Design review of the part built by this model. Coordinates are the model's own, in mm. Face numbers are marked on the shaded views. A direction names the side the tool comes from. Give positions to 0.01 mm unless a question says otherwise; leave off trailing zeros. Write each loop counter-clockwise with the first axis right and the second up, starting at its lowest first coordinate (ties: lowest second). Pieces come first, ordered by that corner, then holes. Notation, with made-up numbers: (17, -31.5) -> (42, -31.5) arc R34 ccw to (42, 6.5) -> close; hole circle Ø4 at (-4.75, -26). An arc over 180 degrees is marked (long way). Return JSON: item names as keys, results as strings. Group by question number.
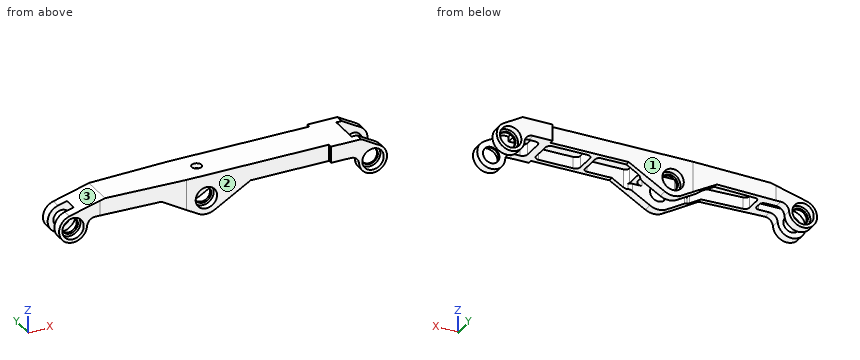
from build123d import *

# Parameters (mm, degrees)
F0_R                   = 5
F1_DEPTH               = 14
F2_W                   = 220
F2_H                   = 50
F3_DEPTH               = 25
F5_DEPTH               = 25
F5_DEPTH_BACK          = 7
F7_DEPTH               = 25
F7_DEPTH_BACK          = 4
F9_DEPTH               = 4
F9_DEPTH_BACK          = 4
F12_DEPTH              = 12
F13_R                  = 2.5
F14_D                  = 6
F18_D                  = 1
F18_DEPTH              = 12
F18_CBORE_D            = 13
F18_CBORE_DEPTH        = 4
F18_TIP                = 0.3004303095
F18_ON_F16_D           = 1
F18_ON_F16_DEPTH       = 12
F18_ON_F16_CBORE_D     = 13
F18_ON_F16_CBORE_DEPTH = 4
F18_ON_F16_TIP         = 0.3004303095
F18_ON_F17_D           = 1
F18_ON_F17_DEPTH       = 12
F18_ON_F17_CBORE_D     = 13
F18_ON_F17_CBORE_DEPTH = 4
F18_ON_F17_TIP         = 0.3004303095
F22_D                  = 1
F22_DEPTH              = 12
F22_CBORE_D            = 13
F22_CBORE_DEPTH        = 4
F22_TIP                = 0.3004303095
F22_ON_F20_D           = 1
F22_ON_F20_DEPTH       = 12
F22_ON_F20_CBORE_D     = 13
F22_ON_F20_CBORE_DEPTH = 4
F22_ON_F20_TIP         = 0.3004303095
F22_ON_F21_D           = 1
F22_ON_F21_DEPTH       = 12
F22_ON_F21_CBORE_D     = 13
F22_ON_F21_CBORE_DEPTH = 4
F22_ON_F21_TIP         = 0.3004303095


with BuildPart() as f1:
    # F0 (on Front) → F1 (new body, symmetric)
    with BuildSketch(Plane.XZ):
        with BuildLine():
            Line((92.751288694, 14), (-60.5927667879, 14))
            Line((-60.5927667879, 14), (-82.1999618834, 8.2103695235))
            ThreePointArc((-82.1999618834, 8.2103695235), (-85.4208481231, -6.5470913868), (-71.5233516925, -0.6296296296))
            ThreePointArc((-71.5233516925, -0.6296296296), (-69.9391570694, 2.664140544), (-66.5370879822, 4))
            Line((-66.5370879822, 4), (-26.9282032303, 4))
            Line((-26.9282032303, 4), (-5, -8.6602540378))
            ThreePointArc((-5, -8.6602540378), (0, -10), (5, -8.6602540378))
            Line((5, -8.6602540378), (26.9282032303, 4))
            Line((26.9282032303, 4), (86.5370879822, 4))
            ThreePointArc((86.5370879822, 4), (89.9391570694, 2.664140544), (91.5233516925, -0.6296296296))
            ThreePointArc((91.5233516925, -0.6296296296), (104.5199051071, -7.1986427765), (104.25, 7.3612159322))
            Line((104.25, 7.3612159322), (92.751288694, 14))
        make_face()
        with Locations((-80, 0)):
            Circle(F0_R, mode=Mode.SUBTRACT)
        Circle(F0_R, mode=Mode.SUBTRACT)
        with Locations((100, 0)):
            Circle(F0_R, mode=Mode.SUBTRACT)
    extrude(amount=F1_DEPTH, both=True)

    # F2 (on face) → F3 (cut)
    with BuildSketch(Plane.XY.offset(14)):
        with Locations((10, 0)):
            Rectangle(F2_W, F2_H)
        Polygon((-63.5, -9.5), (-88.5, -9.5), (-88.5, 9.5), (-63.5, 9.5), (-12, 11.5), (74.5, 11.5), (74.5, 14), (108.5, 14), (108.5, 9), (89.5, 9), (89.5, -9), (108.5, -9), (108.5, -14), (74.5, -14), (74.5, -11.5), (-12, -11.5), align=None, mode=Mode.SUBTRACT)
    extrude(amount=-F3_DEPTH, mode=Mode.SUBTRACT)

    # F4 (on face) → F5 (cut, two sides)
    with BuildSketch(Plane(origin=(0, 0, 4), x_dir=(1, 0, 0), z_dir=(0, 0, -1))) as f5_sk:
        with BuildLine():
            ThreePointArc((74.5, 5.5), (73.6213203436, 7.6213203436), (71.5, 8.5))
            Line((71.5, 8.5), (50.5, 8.5))
            ThreePointArc((50.5, 8.5), (48.3786796564, 7.6213203436), (47.5, 5.5))
            Line((47.5, 5.5), (47.5, -5.5))
            ThreePointArc((47.5, -5.5), (48.3786796564, -7.6213203436), (50.5, -8.5))
            Line((50.5, -8.5), (71.5, -8.5))
            ThreePointArc((71.5, -8.5), (73.6213203436, -7.6213203436), (74.5, -5.5))
            Line((74.5, -5.5), (74.5, 5.5))
        make_face()
        with BuildLine():
            Line((44.5, -6), (44.5, 6))
            ThreePointArc((44.5, 6), (43.767766953, 7.767766953), (42, 8.5))
            Line((42, 8.5), (20, 8.5))
            ThreePointArc((20, 8.5), (18.232233047, 7.767766953), (17.5, 6))
            Line((17.5, 6), (17.5, -6))
            ThreePointArc((17.5, -6), (18.232233047, -7.767766953), (20, -8.5))
            Line((20, -8.5), (42, -8.5))
            ThreePointArc((42, -8.5), (43.767766953, -7.767766953), (44.5, -6))
        make_face()
        with BuildLine():
            Line((89.5, -9), (89.5, 9))
            Line((89.5, 9), (82.5, 9))
            ThreePointArc((82.5, 9), (80.3786796564, 8.1213203436), (79.5, 6))
            Line((79.5, 6), (79.5, -6))
            ThreePointArc((79.5, -6), (80.3786796564, -8.1213203436), (82.5, -9))
            Line((82.5, -9), (89.5, -9))
        make_face()
        with BuildLine():
            Line((-17.5, -5.6851745289), (-17.5, 5.6851745289))
            ThreePointArc((-17.5, 5.6851745289), (-18.2668721376, 7.4869147467), (-20.09701425, 8.1832914668))
            Line((-20.09701425, 8.1832914668), (-52.09701425, 6.9405730202))
            ThreePointArc((-52.09701425, 6.9405730202), (-53.8017402178, 6.1755839447), (-54.5, 4.4424560823))
            Line((-54.5, 4.4424560823), (-54.5, -4.4424560823))
            ThreePointArc((-54.5, -4.4424560823), (-53.8017402178, -6.1755839447), (-52.09701425, -6.9405730202))
            Line((-52.09701425, -6.9405730202), (-20.09701425, -8.1832914668))
            ThreePointArc((-20.09701425, -8.1832914668), (-18.2668721376, -7.4869147467), (-17.5, -5.6851745289))
        make_face()
        with BuildLine():
            Line((-14.5, 1.5), (-14.5, -1.5))
            ThreePointArc((-14.5, -1.5), (-13.1819805153, -4.6819805153), (-10, -6))
            Line((-10, -6), (10, -6))
            ThreePointArc((10, -6), (13.1819805153, -4.6819805153), (14.5, -1.5))
            Line((14.5, -1.5), (14.5, 1.5))
            ThreePointArc((14.5, 1.5), (13.1819805153, 4.6819805153), (10, 6))
            Line((10, 6), (-10, 6))
            ThreePointArc((-10, 6), (-13.1819805153, 4.6819805153), (-14.5, 1.5))
        make_face()
    extrude(amount=F5_DEPTH, mode=Mode.SUBTRACT)
    extrude(f5_sk.sketch, amount=-F5_DEPTH_BACK, mode=Mode.SUBTRACT)

    # F6 (on face) → F7 (cut, two sides)
    with BuildSketch(Plane(origin=(0, 0, 4), x_dir=(1, 0, 0), z_dir=(0, 0, -1))) as f7_sk:
        with BuildLine():
            Line((-88.5, 4), (-88.5, -4))
            Line((-88.5, -4), (-60, -4))
            ThreePointArc((-60, -4), (-58.232233047, -3.267766953), (-57.5, -1.5))
            Line((-57.5, -1.5), (-57.5, 1.5))
            ThreePointArc((-57.5, 1.5), (-58.232233047, 3.267766953), (-60, 4))
            Line((-60, 4), (-88.5, 4))
        make_face()
    extrude(amount=F7_DEPTH, mode=Mode.SUBTRACT)
    extrude(f7_sk.sketch, amount=-F7_DEPTH_BACK, mode=Mode.SUBTRACT)

    # F8 (on Front) → F9 (cut, two sides)
    with BuildSketch(Plane.XZ) as f9_sk:
        with BuildLine():
            Line((-62.9010767594, 1.674937448), (-86.0737760563, 15.0537016249))
            Line((-86.0737760563, 15.0537016249), (-90.8768091461, 6.7346042829))
            Line((-90.8768091461, 6.7346042829), (-84.1196998721, 2.8333854245))
            ThreePointArc((-84.1196998721, 2.8333854245), (-78.5165073914, 4.7748559853), (-75, 0))
            ThreePointArc((-75, 0), (-75.123107113, -1.1026857073), (-75.4863663076, -2.1510720329))
            Line((-75.4863663076, -2.1510720329), (-67.9411956859, -6.5072783225))
            Line((-67.9411956859, -6.5072783225), (-62.9010767594, 1.674937448))
        make_face()
        with BuildLine():
            Line((-75.4863663076, -2.1510720329), (-84.1196998721, 2.8333854245))
            ThreePointArc((-84.1196998721, 2.8333854245), (-82.5, -4.3301270189), (-75.4863663076, -2.1510720329))
        make_face()
        with BuildLine():
            ThreePointArc((-75, 0), (-78.5165073914, 4.7748559853), (-84.1196998721, 2.8333854245))
            Line((-84.1196998721, 2.8333854245), (-75.4863663076, -2.1510720329))
            ThreePointArc((-75.4863663076, -2.1510720329), (-75.123107113, -1.1026857073), (-75, 0))
        make_face()
    extrude(amount=-F9_DEPTH, mode=Mode.SUBTRACT)
    extrude(f9_sk.sketch, amount=F9_DEPTH_BACK, mode=Mode.SUBTRACT)

    # F11 (on offset) → F12 (cut)
    with BuildSketch(Plane.XY.offset(-10)):
        Polygon((-10, -6), (10, -6), (20.6807758659, -6), (20.394064486, 6), (10, 6), (-10, 6), (-21.2499145418, 6), (-20.4144921154, -6), align=None)
    extrude(amount=F12_DEPTH, mode=Mode.SUBTRACT)

    # F13
    f13_edges = [f1.edges().sort_by_distance(p)[0] for p in [
        (-17.519902, -6, 0.284057),
        (17.5, -6, 0.278312),
        (17.5, -6, 6.5),
        (-17.519902, 6, 0.284057),
        (17.5, 6, 0.278312),
        (17.5, 6, 6.5),
    ]]
    fillet(f13_edges, radius=F13_R)

    # F14 (through all)
    with Locations(Plane.XY.offset(14)):
        with Locations((0, 0)):
            Hole(F14_D / 2)

    # F18
    with Locations(Plane.XZ.offset(9.5)):
        with Locations((-80, 0)):
            CounterBoreHole(F18_D / 2, F18_CBORE_D / 2, F18_CBORE_DEPTH, depth=F18_DEPTH)
            with Locations((0, 0, -(F18_DEPTH + F18_TIP / 2))):  # 118° drill point
                Cone(0, F18_D / 2, F18_TIP, mode=Mode.SUBTRACT)

    # F18 on F16
    with Locations(Plane.XZ.offset(11.5)):
        with Locations((0, 0)):
            CounterBoreHole(F18_ON_F16_D / 2, F18_ON_F16_CBORE_D / 2, F18_ON_F16_CBORE_DEPTH, depth=F18_ON_F16_DEPTH)
            with Locations((0, 0, -(F18_ON_F16_DEPTH + F18_ON_F16_TIP / 2))):  # 118° drill point
                Cone(0, F18_ON_F16_D / 2, F18_ON_F16_TIP, mode=Mode.SUBTRACT)

    # F18 on F17
    with Locations(Plane.XZ.offset(14)):
        with Locations((100, 0)):
            CounterBoreHole(F18_ON_F17_D / 2, F18_ON_F17_CBORE_D / 2, F18_ON_F17_CBORE_DEPTH, depth=F18_ON_F17_DEPTH)
            with Locations((0, 0, -(F18_ON_F17_DEPTH + F18_ON_F17_TIP / 2))):  # 118° drill point
                Cone(0, F18_ON_F17_D / 2, F18_ON_F17_TIP, mode=Mode.SUBTRACT)

    # F22
    with Locations(Plane(origin=(0, 14, 0), x_dir=(-1, 0, 0), z_dir=(0, 1, 0))):
        with Locations((-100, 0)):
            CounterBoreHole(F22_D / 2, F22_CBORE_D / 2, F22_CBORE_DEPTH, depth=F22_DEPTH)
            with Locations((0, 0, -(F22_DEPTH + F22_TIP / 2))):  # 118° drill point
                Cone(0, F22_D / 2, F22_TIP, mode=Mode.SUBTRACT)

    # F22 on F20
    with Locations(Plane(origin=(0, 11.5, 0), x_dir=(-1, 0, 0), z_dir=(0, 1, 0))):
        with Locations((0, 0)):
            CounterBoreHole(F22_ON_F20_D / 2, F22_ON_F20_CBORE_D / 2, F22_ON_F20_CBORE_DEPTH, depth=F22_ON_F20_DEPTH)
            with Locations((0, 0, -(F22_ON_F20_DEPTH + F22_ON_F20_TIP / 2))):  # 118° drill point
                Cone(0, F22_ON_F20_D / 2, F22_ON_F20_TIP, mode=Mode.SUBTRACT)

    # F22 on F21
    with Locations(Plane(origin=(0, 9.5, 0), x_dir=(-1, 0, 0), z_dir=(0, 1, 0))):
        with Locations((80, 0)):
            CounterBoreHole(F22_ON_F21_D / 2, F22_ON_F21_CBORE_D / 2, F22_ON_F21_CBORE_DEPTH, depth=F22_ON_F21_DEPTH)
            with Locations((0, 0, -(F22_ON_F21_DEPTH + F22_ON_F21_TIP / 2))):  # 118° drill point
                Cone(0, F22_ON_F21_D / 2, F22_ON_F21_TIP, mode=Mode.SUBTRACT)


solid = f1.part
Q1. Tool access review of the marked faces 1, 2 and 3: name each direction out of +Z, -Z, +X, -X, +Y, -Y from which nothing blocks a thin tool from reaching the whole face with its end or side.
Q2. Take a section at A-A, the plane x = -80. Give the boundary of the cut face in (y, z), plus the area to 3 significant figures.
Q3. For L1, parallel to Y at x = 100.5, z = 5.25; L2, parallel to Y at x = -74.5, z = 6.25; L3, parallel to Z at x = 0, y = 6.45, list the stretches that pass through material, from the lowest coordinate up. Write a range as from..to.
Q4. Insertion check: pin 1 (4 mm diameter, centred on x = 14.5, y = 1.5, fed in from -Z); pin 2 (8 mm diameter, centred on x = 13.5, z = 3, fed in from +Y); pin 3 (3 mm diameter, centred on y = 8.5, z = -6, fed in from +X). Each pin has a flat end and moves straight along its axis. Give the tip position at first contact, or say it passes through.
Q5. Take a section at B-B, the plane x = 100. Give the boundary of the cut face in (y, z).
Final values:
{
 "1": {"face 1": "+Z, -Z, -X, +Y", "face 2": "+Z, -Z, -X, -Y", "face 3": "+Z, -X, +Y, -Y"},
 "2": {"outline": "(-9.5, -8.5) -> (-4, -8.5) -> (-4, -5) -> (-5.5, -5) -> (-5.5, -6.5) -> (-9.5, -6.5) -> close; (-9.5, 6.5) -> (-5.5, 6.5) -> (-5.5, 5) -> (-4, 5) -> (-4, 8.8) -> (-9.5, 8.8) -> close; (4, -8.5) -> (9.5, -8.5) -> (9.5, -6.5) -> (5.5, -6.5) -> (5.5, -5) -> (4, -5) -> close; (4, 5) -> (5.5, 5) -> (5.5, 6.5) -> (9.5, 6.5) -> (9.5, 8.8) -> (4, 8.8) -> close", "area": "56.3 mm²"},
 "3": {"L1": "y = -10..-9, 9..10", "L2": "y = -9.5..-4, 4..9.5", "L3": "z = -10..-5, 5..14"},
 "4": {"pin 1": "stops at z = 2", "pin 2": "stops at y = 11.5", "pin 3": "stops at x = 107.16"},
 "5": {"outline": "(-14, -8.5) -> (-9, -8.5) -> (-9, -5) -> (-10, -5) -> (-10, -6.5) -> (-14, -6.5) -> close; (-14, 6.5) -> (-10, 6.5) -> (-10, 5) -> (-9, 5) -> (-9, 9.81) -> (-14, 9.81) -> close; (9, -8.5) -> (14, -8.5) -> (14, -6.5) -> (10, -6.5) -> (10, -5) -> (9, -5) -> close; (9, 5) -> (10, 5) -> (10, 6.5) -> (14, 6.5) -> (14, 9.81) -> (9, 9.81) -> close"}
}
